Autodesk Fusion 360 part; units mm, degrees
sketch "Sketch1" plane through (0, 0, 0) normal (0, 1, 0) x (1, 0, 0)
  line L0 (0, 0) -> (87, 0)
  line L1 (87, 0) -> (87, 58)
  line L2 (87, 58) -> (0, 58)
  line L3 (0, 58) -> (0, 0)
  line L4 (-3, 61) -> (90, 61)
  line L5 (90, 61) -> (90, -3)
  line L6 (90, -3) -> (-3, -3)
  line L7 (-3, -3) -> (-3, 61)
  dimension "d1" = 87
  dimension "d2" = 58
  dimension "d3" = 3
  dimension "d4" = 3
  dimension "d5" = 3
  dimension "d6" = 3
extrude "Extrude1" add sketch "Sketch1" along normal blind 5
extrude "Extrude2" add sketch "Sketch1" along normal blind 1 contours L0 L1 L2 L3
sketch "Sketch2" plane through (0, 0, 0) normal (0, 1, 0) x (1, 0, 0)
  line L0 (90, -3) -> (-3, -3)
  line L1 (-3, -3) -> (-3, 61)
  line L2 (-3, 61) -> (90, 61)
  line L3 (90, 61) -> (90, -3)
  circle A0 centre (81.6, 63.54) radius 1.75
  circle A1 centre (5.4, 63.54) radius 1.75
  line L4 (-3, -3) -> (-3, 61)
  line L5 (-3, 61) -> (90, 61)
  circle A2 centre (81.6, -5.54) radius 1.75
  circle A3 centre (5.4, -5.54) radius 1.75
  line L6 (90, -3) -> (-3, -3)
  line L7 (-3, 66.08) -> (90, 66.08)
  line L8 (90, 66.08) -> (90, -8.08)
  line L9 (90, -8.08) -> (-3, -8.08)
  line L10 (-3, -8.08) -> (-3, 66.08)
  dimension "d11" = 3.5
  dimension "d12" = 3.5
  dimension "d13" = 76.2
  dimension "d14" = 8.4
  dimension "d15" = 2.54
  dimension "d16" = 3.5
  dimension "d17" = 3.5
  dimension "d18" = 2.54
  dimension "d19" = 2.54
  dimension "d21" = 2.54
  dimension "d22" = 2.54
extrude "Extrude3" add sketch "Sketch2" along normal blind 1.778 contours L0 L6 L8 L9 L10 | L2 L5 L7 L8 L10
equation "d4 = d3"
equation "d5 = d4"
Geometry: final body of the model. Coordinates: model frame, mm. A direction names the side the tool comes from. Coordinates: 2 decimals unless noted, no trailing zeros. Order: outer loops, then holes, each group sorted by start corner. A loop starts at its lowest first (then second) coordinate and runs counter-clockwise, first axis right, second up. Notation, with made-up numbers: (52.5, 79.5) -> (78.5, 79.5) arc R38 ccw to (78.5, 117.5) -> close; hole circle Ø10 at (17, 20.25). An arc over 180 degrees is marked (long way). Answer in a Markdown table with one row per item.
Item 1: Access query for faces 5 (the flat face through (43, 3, -61)), 6 (the flat face through (0, 3, -29)), 7 (the flat face through (-3, 2, -28)), 8 (the flat face through (43, 0, -30)), 9 (the flat face through (43, 1.778, 6)). Directions: +Z, -Z, +X, -X, +Y, -Y. A direction counts if a zero-diameter tool reaches every point of the face in a straight line with its end or side. Return the directions, or none.
Return value:
| item | result |
|---|---|
| face 5 | -Z, +X, -X, +Y |
| face 6 | +Y |
| face 7 | +Z, -Z, -X, +Y, -Y |
| face 8 | +Z, -Z, +X, -X, -Y |
| face 9 | +Z, +X, -X, +Y |
Item 2: Section C-C on y = 2.95. Output: boundary loops of the cut face in (x, z), plus the area to 3 significant figures.
Return value:
| item | result |
|---|---|
| outline | (-3, -61) -> (90, -61) -> (90, 3) -> (-3, 3) -> close; hole (0, -58) -> (87, -58) -> (87, 0) -> (0, 0) -> close |
| area | 906 mm² |
Item 3: Section A-A on x = 5.4. Output: boundary loops of the cut face in (y, z).
Return value:
| item | result |
|---|---|
| outline | (0, -66.08) -> (1.78, -66.08) -> (1.78, -65.29) -> (0, -65.29) -> close; (0, -61.79) -> (1.78, -61.79) -> (1.78, -61) -> (5, -61) -> (5, -58) -> (1, -58) -> (1, 0) -> (5, 0) -> (5, 3) -> (1.78, 3) -> (1.78, 3.79) -> (0, 3.79) -> close; (0, 7.29) -> (1.78, 7.29) -> (1.78, 8.08) -> (0, 8.08) -> close |
Item 4: Ray query, L1, parallel to X at y = 1, z = 5.54; L2, parallel to Z at x = 81.6, y = 1.1; L3, parallel to Z at x = 5.4, y = 0.55. Return the intervals inside material, ascending.
Return value:
| item | result |
|---|---|
| L1 | x = -3 to 3.65, 7.15 to 79.85, 83.35 to 90 |
| L2 | z = -66.08 to -65.29, -61.79 to -58, 0 to 3.79, 7.29 to 8.08 |
| L3 | z = -66.08 to -65.29, -61.79 to 3.79, 7.29 to 8.08 |
Item 5: Draft query along Z for faces 1 (the flat face through (90, 2, -30)), 2 (the flat face through (43, 3, 0)), 3 (the flat face through (87, 3, -29)), 4 (the flat face through (44, 3, 3)). Return one class per face: released by +Z, released by -Z, zero draft, split by the parting line, or undercut.
Return value:
| item | result |
|---|---|
| face 1 | zero draft |
| face 2 | undercut |
| face 3 | undercut |
| face 4 | released by +Z |
Item 6: Section D-D on z = -37. Output: boundary loops of the cut face in (x, y).
Return value:
| item | result |
|---|---|
| outline | (-3, 0) -> (90, 0) -> (90, 5) -> (87, 5) -> (87, 1) -> (0, 1) -> (0, 5) -> (-3, 5) -> close |
Item 7: Contact query for flat-ended pins moving along their axis: P1, Ø1.5, axis at x = 27.5, z = 6.5, coming from the +Y side; P2, Ø3, axis at x = 81.6, z = -63.54, coming from the -Y side; P3, Ø1.6, axis at x = 43.5, y = 3.5, coming from the +Z side; P4, Ø10, axis at x = 80.5, z = -23, coming from the +Y side. Output: stop coordinate, or through.
Return value:
| item | result |
|---|---|
| P1 | stops at y = 1.78 |
| P2 | passes through |
| P3 | stops at z = 3 |
| P4 | stops at y = 1 |
Item 8: Section B-B on z = 5.54. Output: boundary loops of the cut face in (x, y), plus the area to 3 significant figures.
Return value:
| item | result |
|---|---|
| outline | (-3, 0) -> (3.65, 0) -> (3.65, 1.78) -> (-3, 1.78) -> close; (7.15, 0) -> (79.85, 0) -> (79.85, 1.78) -> (7.15, 1.78) -> close; (83.35, 0) -> (90, 0) -> (90, 1.78) -> (83.35, 1.78) -> close |
| area | 153 mm² |
